Design review of the part built by this model. Coordinates are the model's own, in mm. A direction names the side the tool comes from. Coordinates: 2 decimals unless noted, no trailing zeros. Loops run counter-clockwise (first coordinate to the right, second up) from the corner with the lowest first, then second, coordinate; pieces in that order, holes last.
Q1. Machinability: for faces 1 (the face through (16, -14, 0)), 2 (the face through (10, -32.5, -27)), 3 (the face through (6, 18, -1)), which of the approach directions +Z, -Z, +X, -X, +Y, -Y give a long, thin tool a straight path to every point of the face, cutting with its end or side? Answer none if there is none.
Q2. For P1, Ø3, axis at x = 8.5, z = -21.5, coming from the +Y side; P2, Ø8, axis at x = 5, y = 12.5, coming from the -Z side; P3, Ø4.5, axis at x = 10.5, y = 18, coming from the +Z side, all flat-tipped, find the tip position at first contact; note any pin that passes through.
Q3. Wall thickness on probe 1 along X at (y, z) = (-35.75, 25); probe 2 along Y at (x, z) = (0.75, -18); probe 3 along Z at (x, y) = (4.5, 0): over which ranges is each line inside the solid? List them lowest first.
Q4. Add section D-D on z = 10.5. Give the boundary of the cut face in (x, y).
Q5. Add section A-A on x = 8. Give the boundary of the cut face in (y, z).
Q6. Add section C-C on z = -25. Give the boundary of the cut face in (x, y).
Q7. Draft analysis for pull direction Y (two halves, no side actions). For faces 4 (the face through (8, -3, 17.5)), 5 (the face through (5.78, 21.13, -9.37)), 6 (the face through (6, -32.5, 27)), state which applies: released by +Y, released by -Y, zero draft, split by the parting line, or undercut.
Q8. Add section B-B on y = 0. Give the boundary of the cut face in (x, z).
```python
from build123d import *

# Parameters (mm, degrees)
BOSS_EXTRUDE1_DEPTH = 16
SKETCH2_R           = 2.5
CUT_EXTRUDE1_DEPTH  = 71.556714776
SKETCH3_R           = 2.5
CUT_EXTRUDE2_DEPTH  = 68.061538903


with BuildPart() as part:
    # Sketch1 → Boss-Extrude1 (new body)
    with BuildSketch(Plane(origin=(0, 0, 0), x_dir=(0, 0, -1), z_dir=(1, 0, 0))):
        with BuildLine():
            Line((17.5, -32.5), (33.5, -32.5))
            Line((33.5, -32.5), (33.5, -40.5))
            Line((33.5, -40.5), (-33.5, -40.5))
            Line((-33.5, -40.5), (-33.5, -32.5))
            Line((-33.5, -32.5), (-17.5, -32.5))
            Line((-17.5, -32.5), (-17.5, 27.5))
            Line((-17.5, 27.5), (-1, 27.5))
            Line((-1, 27.5), (-1, 12.459935794))
            ThreePointArc((-1, 12.459935794), (0, -12.5), (1, 12.459935794))
            Line((1, 12.459935794), (1, 27.5))
            Line((1, 27.5), (17.5, 27.5))
            Line((17.5, 27.5), (17.5, -32.5))
        make_face()
    extrude(amount=BOSS_EXTRUDE1_DEPTH)

    # Sketch2 → Cut-Extrude1 (cut, through all)
    with BuildSketch(Plane(origin=(0, -32.5, 0), x_dir=(1, 0, 0), z_dir=(0, 1, 0))):
        with Locations(Location((8, -25, 0), (0, 0, 270))):
            Circle(SKETCH2_R)
        with Locations(Location((8, 25, 0), (0, 0, 270))):
            Circle(SKETCH2_R)
    extrude(amount=-CUT_EXTRUDE1_DEPTH, mode=Mode.SUBTRACT)

    # Sketch3 → Cut-Extrude2 (cut, through all)
    with BuildSketch(Plane(origin=(0, 0, -17.5), x_dir=(-1, 0, 0), z_dir=(0, 0, -1))):
        with Locations(Location((-8, 19.979967897, 0), (0, 0, 90))):
            Circle(SKETCH3_R)
    extrude(amount=-CUT_EXTRUDE2_DEPTH, mode=Mode.SUBTRACT)


solid = part.part
```
Entries:
1. face 1: +Z, -Z, +X, +Y, -Y
1. face 2: -Z, +X, -X, +Y
1. face 3: +X, -X, +Y
2. P1: stops at y = -32.5
2. P2: stops at z = -17.5
2. P3: stops at z = 17.5
3. probe 1: x = 0 to 5.5, 10.5 to 16
3. probe 2: y = -40.5 to -32.5
3. probe 3: z = -17.5 to -12.5, 12.5 to 17.5
4. outline: (0, -40.5) - (16, -40.5) - (16, -6.78) - (0, -6.78) - close; (0, 6.78) - (16, 6.78) - (16, 27.5) - (0, 27.5) - close; hole circle Ø5 at (8, 19.98)
5. outline: (-40.5, -33.5) - (-32.5, -33.5) - (-32.5, -27.5) - (-40.5, -27.5) - close; (-40.5, -22.5) - (-32.5, -22.5) - (-32.5, -17.5) - (17.48, -17.5) - (17.48, -1) - (12.46, -1) arc R12.5 cw (long way) to (12.46, 1) - (17.48, 1) - (17.48, 17.5) - (-32.5, 17.5) - (-32.5, 22.5) - (-40.5, 22.5) - close; (-40.5, 27.5) - (-32.5, 27.5) - (-32.5, 33.5) - (-40.5, 33.5) - close; (22.48, -17.5) - (27.5, -17.5) - (27.5, -1) - (22.48, -1) - close; (22.48, 1) - (27.5, 1) - (27.5, 17.5) - (22.48, 17.5) - close
6. outline: (0, -40.5) - (5.5, -40.5) - (5.5, -32.5) - (0, -32.5) - close; (10.5, -40.5) - (16, -40.5) - (16, -32.5) - (10.5, -32.5) - close
7. face 4: zero draft
7. face 5: undercut
7. face 6: released by +Y
8. outline: (0, -17.5) - (16, -17.5) - (16, -12.5) - (0, -12.5) - close; (0, 12.5) - (16, 12.5) - (16, 17.5) - (0, 17.5) - close
